```python
from build123d import *

# Parameters (mm, degrees)
SKETCH1_R                                           = 2.55
BOSS_EXTRUDE1_DEPTH                                 = 3
CBORE_FOR_00_BINDING_HEAD_MACHINE_SCREW_D           = 9.525
CBORE_FOR_00_BINDING_HEAD_MACHINE_SCREW_CBORE_D     = 16.1036
CBORE_FOR_00_BINDING_HEAD_MACHINE_SCREW_CBORE_DEPTH = 1.524


with BuildPart() as part:
    # Sketch1 → Boss-Extrude1 (new body)
    with BuildSketch(Plane(origin=(0, 0, 0), x_dir=(1, 0, 0), z_dir=(0, 1, 0))):
        with BuildLine():
            Line((14.75, -33.5), (-14.75, -33.5))
            ThreePointArc((-14.75, -33.5), (-18.285533906, -32.035533906), (-19.75, -28.5))
            Line((-19.75, -28.5), (-19.75, 28.5))
            ThreePointArc((-19.75, 28.5), (-18.285533906, 32.035533906), (-14.75, 33.5))
            Line((-14.75, 33.5), (14.75, 33.5))
            ThreePointArc((14.75, 33.5), (18.285533906, 32.035533906), (19.75, 28.5))
            Line((19.75, 28.5), (19.75, -28.5))
            ThreePointArc((19.75, -28.5), (18.285533906, -32.035533906), (14.75, -33.5))
        make_face()
        with Locations((0, 26.5)):
            Circle(SKETCH1_R, mode=Mode.SUBTRACT)
        with Locations((10, -25.29)):
            Circle(SKETCH1_R, mode=Mode.SUBTRACT)
        with Locations((10, -5.29)):
            Circle(SKETCH1_R, mode=Mode.SUBTRACT)
        with Locations((0, -25.29)):
            Circle(SKETCH1_R, mode=Mode.SUBTRACT)
        with Locations((0, -5.29)):
            Circle(SKETCH1_R, mode=Mode.SUBTRACT)
        with Locations((-10, -25.29)):
            Circle(SKETCH1_R, mode=Mode.SUBTRACT)
        with Locations((-10, -5.29)):
            Circle(SKETCH1_R, mode=Mode.SUBTRACT)
    extrude(amount=BOSS_EXTRUDE1_DEPTH)

    # CBORE for #00 Binding Head Machine Screw1 (through all)
    with Locations(Plane(origin=(0, 3, 0), x_dir=(1, 0, 0), z_dir=(0, 1, 0))):
        with Locations((0, 22.5)):
            CounterBoreHole(CBORE_FOR_00_BINDING_HEAD_MACHINE_SCREW_D / 2, CBORE_FOR_00_BINDING_HEAD_MACHINE_SCREW_CBORE_D / 2, CBORE_FOR_00_BINDING_HEAD_MACHINE_SCREW_CBORE_DEPTH)


solid = part.part
```
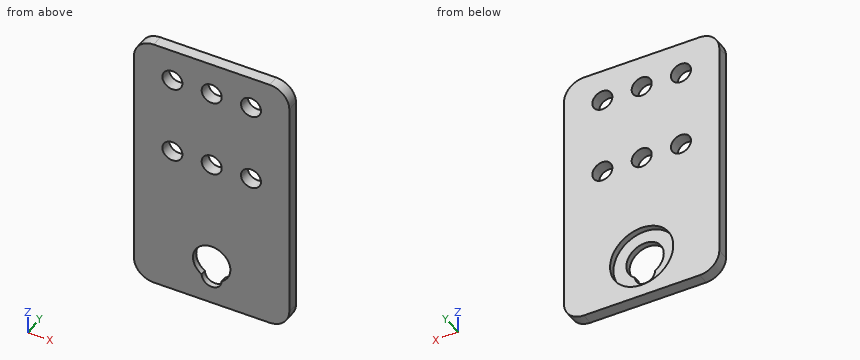
Geometry check sheet. Reference: the model listing, model coordinates, mm. Round coordinates to 2 decimals unless told otherwise and drop trailing zeros. Loops run counter-clockwise (first coordinate to the right, second up) from the corner with the lowest first, then second, coordinate; pieces in that order, holes last. Notation, with made-up numbers: (13.5, -7) - (61.5, -7) arc R8 cw to (61.5, -1) - close; hole circle Ø2 at (44, 61.25). An arc over 180 degrees is marked (long way). Write item = value, one per line. Start each with the question number.
1. Thickness scan on line 1 (X direction, y = 2.1, z = 25.29); line 2 (Z direction, x = 0, y = 2.2); line 3 (Z direction, x = -10, y = 2). Record the ranges inside material, lowest first.
2. Section check A-A on x = 0. Enter the section's corners in (y, z).
3. Section check B-B on z = 5.29. Enter the section's corners in (x, y), then the cut area to 3 significant figures.
4. Depth check by flat-ended pin: pin 1 (8 mm diameter, centred on x = -10, z = 25.29, fed in from +Y); pin 2 (8 mm diameter, centred on x = 1, z = -20.5, fed in from +Y). Enter the tip coordinate at first touch or a pass-through.
5. Section check C-C on y = 2.55. Enter the section's corners in (x, z).
6. Section check D-D on z = -22.5. Enter the section's corners in (x, y), then the cut area to 3 significant figures.
Working result:
q1.line_1 = -19.75 to -12.55, -7.45 to -2.55, 2.55 to 7.45, 12.55 to 19.75
q1.line_2 = -33.5 to -30.55, -14.45 to 2.74, 7.84 to 22.74, 27.84 to 33.5
q1.line_3 = -33.5 to 2.74, 7.84 to 22.74, 27.84 to 33.5
q2.outline = (0, -33.5) - (3, -33.5) - (3, -30.55) - (1.48, -30.55) - (1.48, -29.05) - (0, -29.05) - close; (0, -17.74) - (1.48, -17.74) - (1.48, -14.45) - (3, -14.45) - (3, 2.74) - (0, 2.74) - close; (0, 7.84) - (3, 7.84) - (3, 22.74) - (0, 22.74) - close; (0, 27.84) - (3, 27.84) - (3, 33.5) - (0, 33.5) - close
q3.outline = (-19.75, 0) - (-12.55, 0) - (-12.55, 3) - (-19.75, 3) - close; (-7.45, 0) - (-2.55, 0) - (-2.55, 3) - (-7.45, 3) - close; (2.55, 0) - (7.45, 0) - (7.45, 3) - (2.55, 3) - close; (12.55, 0) - (19.75, 0) - (19.75, 3) - (12.55, 3) - close
q3.area = 72.6 mm^2
q4.pin_1 = 3
q4.pin_2 = 1.48
q5.outline = (-19.75, -28.5) arc R5 ccw to (-14.75, -33.5) - (14.75, -33.5) arc R5 ccw to (19.75, -28.5) - (19.75, 28.5) arc R5 ccw to (14.75, 33.5) - (-14.75, 33.5) arc R5 ccw to (-19.75, 28.5) - close; hole circle Ø5.1 at (-10, 5.29); hole circle Ø5.1 at (-10, 25.29); hole circle Ø16.1 at (0, -22.5); hole circle Ø5.1 at (0, 5.29); hole circle Ø5.1 at (0, 25.29); hole circle Ø5.1 at (10, 5.29); hole circle Ø5.1 at (10, 25.29)
q6.outline = (-19.75, 0) - (-4.76, 0) - (-4.76, 1.48) - (-8.05, 1.48) - (-8.05, 3) - (-19.75, 3) - close; (4.76, 0) - (19.75, 0) - (19.75, 3) - (8.05, 3) - (8.05, 1.48) - (4.76, 1.48) - close
q6.area = 79.9 mm^2
